For this review, take the finished solid that the model builds, in its own axes (mm). A direction names the side the tool comes from. Coordinates: 2 decimals unless noted, no trailing zeros. Write each loop counter-clockwise with the first axis right and the second up, starting at its lowest first coordinate (ties: lowest second). Pieces come first, ordered by that corner, then holes. Notation, with made-up numbers: (42, 66) -> (56, 66) arc R5 ccw to (56, 71) -> close; hole circle Ø6 at (29, 47). An arc over 180 degrees is marked (long way). Put each result on its own line as item: value. Start each with the question number.
Item 1: To check wall thickness, follow L1, parallel to Y at x = 15.75, z = 0; L2, parallel to Y at x = 10.75, z = 0; L3, parallel to Y at x = 8, z = 31. State the ranges of each line that lie inside material, in increasing order.
Item 2: For faces 1 (the cylindrical face through (4.733, -34.717, 1.774)), 2 (the cylindrical face through (12.304, 9.782, 21.938)), 3 (the cylindrical face through (3.465, -19.524, -4.336)), list the 3-axis set-ups (+Z, -Z, +X, -X, +Y, -Y) from which the entire face can be reached by the end or side of a thin tool; tool diameter is ignored.
Item 3: Consider section A-A on y = -37.5. Give the boundary of the cut face in (x, z) (3 decimals).
Item 4: Insertion check: P1, Ø6, axis at x = 10, y = 20.5, coming from the +Z side; P2, Ø2, axis at y = -18, z = 2, coming from the -X side; P3, Ø6.5, axis at y = 12, z = 20.78, coming from the +X side. Each pin has a flat end and moves straight along its axis. Give the tip position at first contact, or say it passes through.
Item 5: Consider section B-B on x = 2.75. Give the boundary of the cut face in (y, z), and give its area (3 significant figures).
Item 6: The part is to be moulded in two halves that separate along Y. For faces 4 (the flat face through (9, -9, 29)), 5 (the cylindrical face through (13.06, 1.32, -29.97)), 6 (the conical face through (5.667, 34.53, -1.894)), say which applies: +Y half, -Y half, draft (parallel to the pull), parting line (faces both ways), or undercut.
```python
from build123d import *

# Parameters (mm, degrees)
PATTERN_CIRCULAR_1_COUNT = 6
PATTERN_CIRCULAR_2_COUNT = 6
CUT_EXTRUDE_START        = -4
SKETCH_8_R               = 18
SKETCH_8_R_2             = 15
CUT_EXTRUDE_1_DEPTH      = 4
CHAMFER_1_SIZE           = 1
CHAMFER_2_SIZE           = 1


with BuildPart() as part:
    # Эскиз1 → Повернуть1 (revolve)
    with BuildSketch(Plane.XY, mode=Mode.PRIVATE) as revolve_1_sk:
        Polygon((0, 20), (0, 27.5), (4, 27.5), (4, 45), (9, 45), (9, 30), (17, 30), (17, 15), (6, 15), (6, 20), align=None)
    revolve(revolve_1_sk.sketch.rotate(Axis((0, 0, 0), (-1, 0, 0)), 270), axis=Axis((0, 0, 0), (-1, 0, 0)))

    # Эскиз3 → Hole Wizard M61 (revolve, cut)
    with BuildSketch(Plane(origin=(17, 24, 0), x_dir=(0, 0, -1), z_dir=(0, 1, 0))):
        Polygon((0, 0), (0, 10), (2.5, 8.497848452), (2.5, 0), align=None)
    hole_wizard_m61 = revolve(axis=Axis((23.35, 24, 0), (-1, 0, 0)), mode=Mode.SUBTRACT)

    # Круговой массив1: Hole Wizard M61 ×6 about axis
    pattern_circular_1_axis = Axis((0, 0, 0), (1, 0, 0))
    for i in range(1, PATTERN_CIRCULAR_1_COUNT):
        add(hole_wizard_m61.rotate(pattern_circular_1_axis, i * 360 / PATTERN_CIRCULAR_1_COUNT), mode=Mode.SUBTRACT)

    # Эскиз6 → Hole Wizard M61 2 (revolve, cut)
    with BuildSketch(Plane(origin=(9, 37.5, 0), x_dir=(0, 0, -1), z_dir=(0, 1, 0))):
        Polygon((0, 0), (0, 13), (3.3, 11.017159957), (3.3, 3.555), (6.855, 0), align=None)
    hole_wizard_m61_2 = revolve(axis=Axis((15.35, 37.5, 0), (-1, 0, 0)), mode=Mode.SUBTRACT)

    # Круговой массив2: Hole Wizard M61 2 ×6 about axis
    pattern_circular_2_axis = Axis((0, 0, 0), (1, 0, 0))
    for i in range(1, PATTERN_CIRCULAR_2_COUNT):
        add(hole_wizard_m61_2.rotate(pattern_circular_2_axis, i * 360 / PATTERN_CIRCULAR_2_COUNT), mode=Mode.SUBTRACT)

    # Эскиз8 → Вырез-Вытянуть1 (cut)
    with BuildSketch(Plane(origin=(17, 0, 0), x_dir=(0, 0, -1), z_dir=(1, 0, 0)).offset(CUT_EXTRUDE_START)):
        Circle(SKETCH_8_R)
        with Locations(Location((0, 0, 0), (0, 0, 180))):
            Circle(SKETCH_8_R_2, mode=Mode.SUBTRACT)
    extrude(amount=CUT_EXTRUDE_1_DEPTH, mode=Mode.SUBTRACT)

    # Фаска1
    chamfer_1_edges = [part.edges().sort_by_distance(p)[0] for p in [
        (17, 24, 2.5),
        (17, 14.165063509, -19.534609691),
        (17, -9.834936491, -22.034609691),
        (17, -24, -2.5),
        (17, -14.165063509, 19.534609691),
        (17, 9.834936491, 22.034609691),
    ]]
    chamfer(chamfer_1_edges, length=CHAMFER_1_SIZE)

    # Фаска2
    chamfer_2_edges = [part.edges().sort_by_distance(p)[0] for p in [
        (17, 0, 18),
        (0, 0, -27.5),
        (0, 0, -20),
    ]]
    chamfer(chamfer_2_edges, length=CHAMFER_2_SIZE)


solid = part.part
```
Return value:
1. L1: -30 to -26.5, -21.5 to -18, 18 to 21.5, 26.5 to 30
1. L2: -30 to -26.5, -21.5 to -15, 15 to 21.5, 26.5 to 30
1. L3: -32.62 to -24.42, -13.08 to 13.08, 24.42 to 32.62
2. face 1: +X, -X
2. face 2: +X
2. face 3: -X
3. outline: (4, -24.875) -> (9, -24.875) -> (9, -6.855) -> (5.445, -3.3) -> (4, -3.3) -> close; (4, 3.3) -> (5.445, 3.3) -> (9, 6.855) -> (9, 24.875) -> (4, 24.875) -> close
4. P1: z = 41.38
4. P2: x = 6
4. P3: x = 16.75
5. outline: circle Ø55 at (0, 0); hole circle Ø40 at (0, 0)
5. area: 1,120 mm^2
6. face 4: draft
6. face 5: parting line
6. face 6: undercut
